Input: part model. Units: mm. Frame: model coordinates. Face numbers are marked on the shaded views. A direction names the side the tool comes from. Coordinates: 2 decimals unless noted, no trailing zeros. Loops run counter-clockwise (first coordinate to the right, second up) from the corner with the lowest first, then second, coordinate; pieces in that order, holes last.
Autodesk Inventor part; units mm, degrees
ref_plane "YZ Plane" through (0, 0, 0) normal (1, 0, 0) x (0, 1, 0)
ref_plane "XZ Plane" through (0, 0, 0) normal (0, 1, 0) x (-1, 0, 0)
ref_plane "XY Plane" through (0, 0, 0) normal (0, 0, 1) x (1, 0, 0)
sketch "Sketch1" plane through (0, 0, 0) normal (0, 0, 1) x (1, 0, 0)
  line L0 (-17.386, 3.6293) -> (12.614, 3.6293)
  line L1 (12.614, 3.6293) -> (12.614, -9.6107)
  line L2 (12.614, -9.6107) -> (-17.386, -9.6107)
  line L3 (-17.386, -9.6107) -> (-17.386, 3.6293)
  point P0 (0, 0)
  dimension "d0" = 30
  dimension "d1" = 13.24
extrude "Extrusion1" add sketch "Sketch1" along normal blind 5
sketch "Sketch5" plane through (0, 0, 5) normal (0, 0, 1) x (1, 0, 0)
  line L0 (-9.3427, 3.6227) -> (3.8907, -9.6107)
  line L1 (-4.7873, 3.6293) -> (8.4461, -9.6041)
  line L2 (-4.7873, 3.6293) -> (13.9275, 3.6293) construction
  line L3 (-9.3427, 3.6227) -> (-9.3427, -9.6107)
  line L4 (-9.3427, -9.6107) -> (3.8907, -9.6107)
  line L5 (3.8907, -9.6107) -> (3.8907, -9.6107)
  line L6 (-4.7873, 3.6293) -> (9.938, 3.6293)
  line L7 (12.614, 3.6293) -> (-17.386, 3.6293)
  line L8 (9.938, 3.6293) -> (9.938, -9.6107)
  line L9 (-17.386, -9.6107) -> (12.614, -9.6107)
  line L10 (8.4461, -9.6041) -> (9.938, -9.6107)
  line L11 (-9.3427, 3.6227) -> (-9.3427, -9.6107)
  line L12 (3.8907, -9.6107) -> (-9.3427, -9.6107)
  line L13 (3.8907, -9.6107) -> (-9.3427, 3.6227)
  line L14 (-4.7873, 3.6293) -> (8.4461, -9.6041)
  line L15 (8.4461, -9.6041) -> (9.938, -9.6107)
  line L16 (9.938, 3.6293) -> (9.938, -9.6107)
  line L17 (9.938, 3.6293) -> (-4.7873, 3.6293)
  point P0 (0, 0)
  dimension "d15" = 45
  dimension "d16" = 3.2258
  dimension "d17" = 13.2334
  dimension "d18" = 18.7148
  dimension "d19" = 18.7148
extrude "Extrusion5" add sketch "Sketch5" along normal blind 1.8
sketch "Sketch6" plane through (0, 0, 6.8) normal (0, 0, 1) x (1, 0, 0)
  line L0 (9.938, 3.6293) -> (-4.7873, 3.6293)
  line L1 (12.614, -9.6107) -> (-17.386, -9.6107)
  line L2 (-1.4744, 3.6293) -> (1.6007, 3.6293)
  line L3 (1.6007, 3.6293) -> (1.6007, -9.6107)
  line L4 (1.6007, -9.6107) -> (-1.4744, -9.6107)
  line L5 (-1.4744, -9.6107) -> (-1.4744, 3.6293)
  point P0 (0, 0)
extrude "Extrusion6" add sketch "Sketch6" along normal blind 6.2
sketch "Sketch9" plane through (0, 0, 13) normal (0, 0, 1) x (1, 0, 0)
  line L0 (-1.4744, -4.2456) -> (-9.3427, 3.6227)
  line L1 (-9.3427, 3.6227) -> (3.8907, -9.6107)
  line L2 (-1.4744, -4.2456) -> (3.8907, -9.6107)
  line L3 (3.8907, -9.6107) -> (3.8907, -5.0487)
  line L4 (8.4461, -9.6041) -> (-4.7873, 3.6293)
  line L5 (3.8907, -5.0487) -> (-2.9105, 1.7525)
  line L6 (-2.9105, 1.7525) -> (-2.9105, -2.8095)
  line L7 (-1.4744, -4.2456) -> (-2.9105, -2.8095)
  point P0 (0, 0)
extrude "Extrusion7" cut sketch "Sketch9" against normal blind 6.3
sketch "Sketch10" plane through (0, 0, 13) normal (0, 0, 1) x (1, 0, 0)
  line L0 (12.614, -9.6107) -> (-17.386, -9.6107)
  line L1 (1.6007, 3.6293) -> (-1.4744, 3.6293)
  line L2 (-0.1, -9.6107) -> (0.1, -9.6107)
  line L3 (0.1, -9.6107) -> (0.1, 3.6293)
  line L4 (0.1, 3.6293) -> (-0.1, 3.6293)
  line L5 (-0.1, 3.6293) -> (-0.1, -9.6107)
  line L6 (0, -6.9346) -> (0, -6.5072) construction
  point P0 (0, 0)
  dimension "d26" = 0.2
extrude "Extrusion8" cut sketch "Sketch10" against normal blind 10
sketch "Sketch11" plane through (0, 0, 5) normal (0, 0, 1) x (1, 0, 0)
  line L0 (9.938, 3.6293) -> (1.6007, 3.6293)
  line L1 (9.938, -9.6107) -> (12.614, -9.6107)
  line L2 (9.938, 3.6293) -> (12.614, 3.6293)
  line L3 (12.614, 3.6293) -> (12.614, -9.6107)
  line L4 (12.614, -9.6107) -> (9.938, -9.6107)
  line L5 (9.938, -9.6107) -> (9.938, 3.6293)
  line L6 (-17.386, -9.6107) -> (-9.3427, -9.6107)
  line L7 (-9.3427, 3.6227) -> (-9.3427, -9.6107)
  line L8 (-17.386, -9.6107) -> (-9.3427, -9.6107)
  line L9 (-9.3427, -9.6107) -> (-9.3427, 3.6227)
  line L10 (-9.3427, 3.6227) -> (-17.386, 3.6227)
  line L11 (-17.386, 3.6227) -> (-17.386, -9.6107)
  point P0 (0, 0)
extrude "Extrusion9" add sketch "Sketch11" along normal blind 1.8034
properties part number "BalsaBoi2"
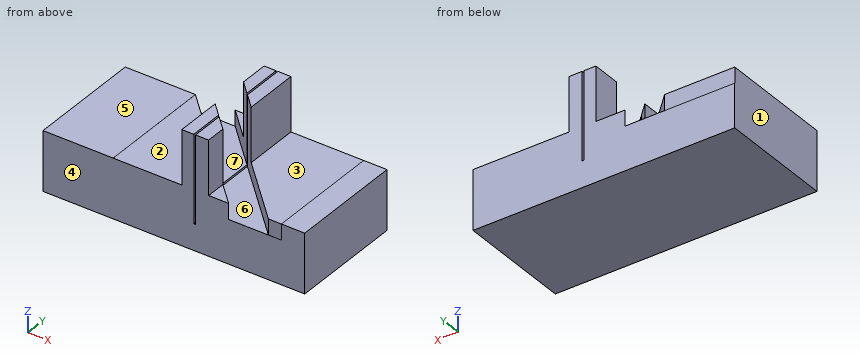
Item 1: Mould query, pull axis Y, two halves, no side actions, for the marked faces 4, 5, 6 and 7. Classes: +Y half, -Y half, draft (parallel to the pull), parting line (faces both ways), or undercut.
Result:
face 4: -Y half
face 5: draft
face 6: undercut
face 7: undercut
Item 2: Line query: L1, parallel to X at y = -6.5, z = 3.25; L2, parallel to X at y = 1.25, z = 9.75; L3, parallel to Z at x = 2.5, y = 1.75. Output: solid intervals per line, ascending.
Result:
L1: x = -17.39 to -0.1, 0.1 to 12.61
L2: x = -1.47 to -0.1, 0.1 to 1.6
L3: z = 0 to 6.8
Item 3: Section query B-B (x = -8.5). Output: boundary loops of the cut face in (y, z).
Result:
outline: (-9.61, 0) - (3.63, 0) - (3.63, 5) - (2.78, 5) - (2.78, 6.8) - (-9.61, 6.8) - close
Item 4: Contact query for flat-ended pins moving along their axis: P1, Ø1, axis at y = 1.5, z = 9.5, coming from the -X side; P2, Ø2, axis at x = 11, y = -3.5, coming from the +Z side; P3, Ø3, axis at y = 0, z = 10.5, coming from the +X side. Output: stop coordinate, or through.
Result:
P1: stops at x = -1.47
P2: stops at z = 6.8
P3: stops at x = 1.6
Item 5: Reachability of the marked faces 1, 2 and 3 from +Z, -Z, +X, -X, +Y, -Y: full face, straight path, thin tool, end or side. Return the list, or none.
Result:
face 1: +Z, -Z, -X, +Y, -Y
face 2: +Z, -X, +Y, -Y
face 3: +Z, +X, +Y, -Y
Item 6: Section query A-A (z = 6.5). Output: boundary loops of the cut face in (x, y).
Result:
outline: (-17.39, -9.61) - (-0.1, -9.61) - (-0.1, -5.62) - (-9.34, 3.62) - (-17.39, 3.62) - close; (-4.79, 3.63) - (-0.1, -1.06) - (-0.1, 3.63) - close; (0.1, -9.61) - (3.89, -9.61) - (0.1, -5.82) - close; (0.1, -1.26) - (8.45, -9.6) - (9.94, -9.61) - (12.61, -9.61) - (12.61, 3.63) - (0.1, 3.63) - close
